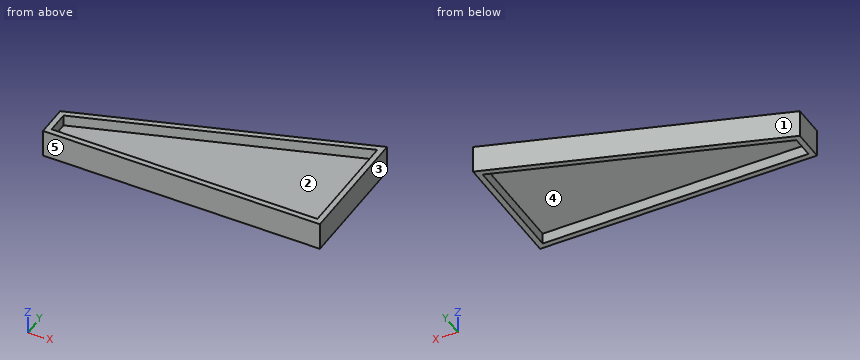
from build123d import *

# Parameters (mm, degrees)
BOSS_EXTRUDE1_DEPTH      = 12.7
BOSS_EXTRUDE2_DEPTH      = 25.4
BOSS_EXTRUDE2_DEPTH_BACK = 38.1


with BuildPart() as part:
    # Sketch1 → Boss-Extrude1 (new body)
    with BuildSketch(Plane.XY):
        Polygon((0, 0), (0, 254), (-609.6, 50.8), (-609.6, 0), align=None)
    extrude(amount=BOSS_EXTRUDE1_DEPTH)

    # Sketch2 → Boss-Extrude2 (add, two sides)
    with BuildSketch(Plane.XY.offset(12.7)) as boss_extrude2_sk:
        Polygon((12.7, -12.7), (12.7, 271.620308761), (-622.3, 59.953642095), (-622.3, -12.7), align=None)
        Polygon((0, 254), (-609.6, 50.8), (-609.6, 0), (0, 0), align=None, mode=Mode.SUBTRACT)
    extrude(amount=BOSS_EXTRUDE2_DEPTH)
    extrude(boss_extrude2_sk.sketch, amount=-BOSS_EXTRUDE2_DEPTH_BACK)


solid = part.part
Verification items for the finished model (mm, model axes). Face numbers are marked on the shaded views. A direction names the side the tool comes from. Give positions to 0.01 mm unless a question says otherwise; leave off trailing zeros. Loops run counter-clockwise (first coordinate to the right, second up) from the corner with the lowest first, then second, coordinate; pieces in that order, holes last.
1) Sectioned sample at C-C, the plane x = -525. Enter the section's corners in (y, z).
2) Set-up check for the marked faces 1 and 2: record each of +Z, -Z, +X, -X, +Y, -Y from which the full face is reachable in a straight line by a thin tool's end or side.
3) Thickness scan on line 1 along Z through (x, y) = (-446, 25.5); line 2 along Y through (x, z) = (-377, 25.5); line 3 along Y through (x, z) = (-202.5, 29.5). Record the ranges inside material, lowest first.
4) Sectioned sample at A-A, the plane z = 32. Enter the section's corners in (x, y), then the cut area to 3 significant figures.
5) Sectioned sample at B-B, the plane y = 104. Enter the section's corners in (x, z), then the cut area to 3 significant figures.
6) Draft check along Y on the marked faces 3, 4 and 5. Enter one of: pulls with the +Y half, pulls with the -Y half, needs draft (parallel to the pull), parting line crosses it, or undercut.
7) Sectioned sample at D-D, the plane z = 6.5. Enter the section's corners in (x, y).
8) Depth check by flat-ended pin: pin 1 Ø1 at (x, z) = (-480.5, 30) entering from +Y; pin 2 Ø1 at (x, z) = (-204, 1.5) entering from +Y; pin 3 Ø8 at (x, y) = (-74, 165.5) entering from +Z. Enter the tip coordinate at first touch or a pass-through.
Answers:
1. outline: (-12.7, -25.4) - (0, -25.4) - (0, 0) - (79, 0) - (79, -25.4) - (92.39, -25.4) - (92.39, 38.1) - (79, 38.1) - (79, 12.7) - (0, 12.7) - (0, 38.1) - (-12.7, 38.1) - close
2. face 1: +Z, -Z, -X, +Y
2. face 2: +Z
3. line 1: z = 0 to 12.7
3. line 2: y = -12.7 to 0, 128.33 to 141.72
3. line 3: y = -12.7 to 0, 186.5 to 199.89
4. outline: (-622.3, -12.7) - (12.7, -12.7) - (12.7, 271.62) - (-622.3, 59.95) - close; hole (-609.6, 0) - (0, 0) - (0, 254) - (-609.6, 50.8) - close
4. area: 20,400 mm2
5. outline: (-490.16, -25.4) - (-450, -25.4) - (-450, 0) - (0, 0) - (0, -25.4) - (12.7, -25.4) - (12.7, 38.1) - (0, 38.1) - (0, 12.7) - (-450, 12.7) - (-450, 38.1) - (-490.16, 38.1) - close
5. area: 9,070 mm2
6. face 3: needs draft
6. face 4: undercut
6. face 5: pulls with the -Y half
7. outline: (-622.3, -12.7) - (12.7, -12.7) - (12.7, 271.62) - (-622.3, 59.95) - close
8. pin 1: stops at y = 107.39
8. pin 2: stops at y = 199.55
8. pin 3: stops at z = 12.7
